Could you check a few things on this model? Use its own coordinates, in mm. A direction names the side the tool comes from. Round coordinates to 2 decimals unless told otherwise and drop trailing zeros. Write each loop counter-clockwise with the first axis right and the second up, starting at its lowest first coordinate (ties: lowest second). Pieces come first, ordered by that corner, then holes. Notation, with made-up numbers: (65, -32) -> (78, -32) arc R13 cw to (78, -16) -> close; hole circle Ø8 at (24.25, 60). An arc over 180 degrees is marked (long way). Return JSON: item names as keys, results as strings.
from build123d import *

# Parameters (mm, degrees)
SKETCH1_W                  = 114
SKETCH1_H                  = 125
BOSS_EXTRUDE1_DEPTH        = 65
SKETCH2_W                  = 111.6
SKETCH2_H                  = 122.6
CUT_EXTRUDE1_DEPTH         = 63.8
SKETCH3_W                  = 44
SKETCH3_H                  = 22
BOSS_EXTRUDE2_DEPTH        = 5
SKETCH4_W                  = 2.65
SKETCH4_H                  = 15
CUT_EXTRUDE2_DEPTH         = 4
SKETCH6_W                  = 2.65
SKETCH6_H                  = 15
CUT_EXTRUDE3_DEPTH         = 4
FILLET1_R                  = 15
FILLET2_R                  = 15
SKETCH9_W                  = 111.6
SKETCH9_H                  = 57.6
SKETCH9_W_2                = 48.6
SKETCH9_H_2                = 48.6
SKETCH9_W_3                = 53.6
SKETCH9_H_3                = 53.6
BOSS_EXTRUDE4_DEPTH        = 9
SKETCH10_W                 = 111.6
SKETCH10_H                 = 56.8
SKETCH10_W_2               = 47
SKETCH10_H_2               = 47
SKETCH10_W_3               = 52
SKETCH10_H_3               = 52
CUT_EXTRUDE5_DEPTH         = 9
SKETCH11_W                 = 4.5
SKETCH11_H                 = 4.5
SKETCH11_H_2               = 56.8
BOSS_EXTRUDE5_DEPTH        = 6
SKETCH12_W                 = 10
SKETCH12_H                 = 5
BOSS_EXTRUDE6_DEPTH        = 5
CHAMFER1_SIZE              = 9
CHAMFER1_SIZE_2            = 5.196152423
CHAMFER1_OF_MIRROR8_SIZE   = 9
CHAMFER1_OF_MIRROR8_SIZE_2 = 5.196152423


with BuildPart() as part:
    # Sketch1 → Boss-Extrude1 (new body)
    with BuildSketch(Plane(origin=(0, 0, 0), x_dir=(1, 0, 0), z_dir=(0, 1, 0))):
        Rectangle(SKETCH1_W, SKETCH1_H)
    extrude(amount=BOSS_EXTRUDE1_DEPTH)

    # Sketch2 → Cut-Extrude1 (cut)
    with BuildSketch(Plane(origin=(0, 65, 0), x_dir=(1, 0, 0), z_dir=(0, 1, 0))):
        Rectangle(SKETCH2_W, SKETCH2_H)
    extrude(amount=-CUT_EXTRUDE1_DEPTH, mode=Mode.SUBTRACT)

    # Sketch3 → Boss-Extrude2 (add)
    with BuildSketch(Plane(origin=(57, 0, 0), x_dir=(0, 0, -1), z_dir=(1, 0, 0))):
        with Locations((-17.5, 44)):
            Rectangle(SKETCH3_W, SKETCH3_H)
    boss_extrude2 = extrude(amount=BOSS_EXTRUDE2_DEPTH)

    # Sketch4 → Cut-Extrude2 (cut)
    with BuildSketch(Plane.XY.offset(39.5)):
        with Locations((58.325, 40.5)):
            Rectangle(SKETCH4_W, SKETCH4_H)
    cut_extrude2 = extrude(amount=-CUT_EXTRUDE2_DEPTH, mode=Mode.SUBTRACT)

    # Sketch6 → Cut-Extrude3 (cut)
    with BuildSketch(Plane(origin=(0, 0, -4.5), x_dir=(-1, 0, 0), z_dir=(0, 0, -1))):
        with Locations((-58.325, 40.5)):
            Rectangle(SKETCH6_W, SKETCH6_H)
    cut_extrude3 = extrude(amount=-CUT_EXTRUDE3_DEPTH, mode=Mode.SUBTRACT)

    # Mirror5: Boss-Extrude2 across plane
    add(boss_extrude2.mirror(Plane(origin=(0, 0, 0), x_dir=(0, 0, 1), z_dir=(1, 0, 0))))

    # Mirror6: Cut-Extrude2 across plane
    add(cut_extrude2.mirror(Plane(origin=(0, 0, 0), x_dir=(0, 0, 1), z_dir=(1, 0, 0))), mode=Mode.SUBTRACT)

    # Mirror7: Cut-Extrude3 across plane
    add(cut_extrude3.mirror(Plane(origin=(0, 0, 0), x_dir=(0, 0, 1), z_dir=(1, 0, 0))), mode=Mode.SUBTRACT)

    # Fillet1
    # the kernel refuses this fillet: 15 mm, written as the material it takes off along each edge
    with BuildSketch(Plane(origin=(62, 33, -32.450849719), x_dir=(-1, 0, 0), z_dir=(0, 0, 1))) as fillet1_piece_1:
        with BuildLine():
            CenterArc((15, -11.180339887), FILLET1_R, 131.810314896, 48.189685104)
            Line((0, -11.180339887), (-0.3, -11.180339887))
            Line((-0.3, -11.180339887), (-0.3, 0))
            Line((-0.3, 0), (0, 0.3))
            ThreePointArc((0, 0.3), (2.5, 0.3), (4.8, 0.223606798))
            Line((4.8, 0.223606798), (5, 0))
        make_face()
    extrude(amount=99.901699437, mode=Mode.SUBTRACT)

    # Fillet2
    # the kernel refuses this fillet: 15 mm, written as the material it takes off along each edge
    with BuildSketch(Plane(origin=(-62, 33, -32.450849719), x_dir=(1, 0, 0), z_dir=(0, 0, 1))) as fillet2_piece_1:
        with BuildLine():
            CenterArc((15, 11.180339887), FILLET2_R, 180, 48.189685104)
            Line((0, 11.180339887), (-0.3, 11.180339887))
            Line((-0.3, 11.180339887), (-0.3, 0))
            Line((-0.3, 0), (0, -0.3))
            ThreePointArc((0, -0.3), (2.5, -0.3), (4.8, -0.223606798))
            Line((4.8, -0.223606798), (5, 0))
        make_face()
    extrude(amount=99.901699437, mode=Mode.SUBTRACT)

    # Sketch9 → Boss-Extrude4 (add)
    with BuildSketch(Plane(origin=(0, 1.2, 0), x_dir=(1, 0, 0), z_dir=(0, 1, 0))):
        with Locations((0, 32.5)):
            Rectangle(SKETCH9_W, SKETCH9_H)
        with Locations((-27.5, -33)):
            Rectangle(SKETCH9_W_2, SKETCH9_H_2)
        with Locations((25, -30.5)):
            Rectangle(SKETCH9_W_3, SKETCH9_H_3)
    extrude(amount=BOSS_EXTRUDE4_DEPTH)

    # Sketch10 → Cut-Extrude5 (cut)
    with BuildSketch(Plane(origin=(0, 10.2, 0), x_dir=(1, 0, 0), z_dir=(0, 1, 0))):
        with Locations((0, 32.9)):
            Rectangle(SKETCH10_W, SKETCH10_H)
        with Locations((-27.5, -33)):
            Rectangle(SKETCH10_W_2, SKETCH10_H_2)
        with Locations((25, -30.5)):
            Rectangle(SKETCH10_W_3, SKETCH10_H_3)
    extrude(amount=-CUT_EXTRUDE5_DEPTH, mode=Mode.SUBTRACT)

    # Sketch11 → Boss-Extrude5 (add)
    with BuildSketch(Plane(origin=(0, 1.2, 0), x_dir=(1, 0, 0), z_dir=(0, 1, 0))):
        with Locations((-53.55, 59.05)):
            Rectangle(SKETCH11_W, SKETCH11_H)
        with Locations((-53.55, 6.75)):
            Rectangle(SKETCH11_W, SKETCH11_H)
        with Locations((53.55, 32.9)):
            Rectangle(SKETCH11_W, SKETCH11_H_2)
        with Locations((-48.75, -11.75)):
            Rectangle(SKETCH11_W, SKETCH11_H)
        with Locations((1.25, -6.75)):
            Rectangle(SKETCH11_W, SKETCH11_H)
        with Locations((-6.25, -11.75)):
            Rectangle(SKETCH11_W, SKETCH11_H)
        with Locations((48.75, -6.75)):
            Rectangle(SKETCH11_W, SKETCH11_H)
        with Locations((-48.75, -54.25)):
            Rectangle(SKETCH11_W, SKETCH11_H)
        with Locations((1.25, -54.25)):
            Rectangle(SKETCH11_W, SKETCH11_H)
        with Locations((-6.25, -54.25)):
            Rectangle(SKETCH11_W, SKETCH11_H)
        with Locations((48.75, -54.25)):
            Rectangle(SKETCH11_W, SKETCH11_H)
        with Locations((0, 32.9)):
            Rectangle(SKETCH11_W, SKETCH11_H)
    extrude(amount=BOSS_EXTRUDE5_DEPTH)

    # Sketch12 → Boss-Extrude6 (add)
    with BuildSketch(Plane.ZY.offset(-55.8)):
        with Locations((-36.3, 34.7)):
            Rectangle(SKETCH12_W, SKETCH12_H)
        with Locations((36.3, 34.7)):
            Rectangle(SKETCH12_W, SKETCH12_H)
    boss_extrude6 = extrude(amount=BOSS_EXTRUDE6_DEPTH)

    # Chamfer1
    # the kernel refuses this chamfer: 9, 5.196152423 mm, written as the material it adds along each edge
    with BuildSketch(Plane(origin=(55.8, 32.2, 41.3), x_dir=(0.019326765612700678, -0.999813220622208, 0), z_dir=(0, 0, -1))) as chamfer1_piece_1_section:
        Polygon((CHAMFER1_SIZE * 0.999813220622, CHAMFER1_SIZE * 0.0193267656127), (-CHAMFER1_SIZE_2 * 0.0193267656116, CHAMFER1_SIZE_2 * 0.999813220566), (0, 0), align=None)
    chamfer1_piece_1 = extrude(amount=10, mode=Mode.PRIVATE)
    chamfer1_piece_1 = split(chamfer1_piece_1, bisect_by=Plane(origin=(50.8, 29.159896695, 36.3), z_dir=(1, 0, 0)), keep=Keep.TOP, mode=Mode.PRIVATE)
    add(chamfer1_piece_1)
    with BuildSketch(Plane(origin=(55.8, 32.2, -31.3), x_dir=(0.019326765612700678, -0.999813220622208, 0), z_dir=(0, 0, -1))) as chamfer1_piece_2_section:
        Polygon((CHAMFER1_SIZE * 0.999813220622, CHAMFER1_SIZE * 0.0193267656127), (-CHAMFER1_SIZE_2 * 0.0193267656116, CHAMFER1_SIZE_2 * 0.999813220566), (0, 0), align=None)
    chamfer1_piece_2 = extrude(amount=10, mode=Mode.PRIVATE)
    chamfer1_piece_2 = split(chamfer1_piece_2, bisect_by=Plane(origin=(50.8, 29.159896695, -36.3), z_dir=(1, 0, 0)), keep=Keep.TOP, mode=Mode.PRIVATE)
    add(chamfer1_piece_2)

    # Mirror8: Boss-Extrude6 across plane
    add(boss_extrude6.mirror(Plane(origin=(0, 0, 0), x_dir=(0, 0, 1), z_dir=(1, 0, 0))))

    # Chamfer1 of Mirror8
    # the kernel refuses this chamfer: 9, 5.196152423 mm, written as the material it adds along each edge
    with BuildSketch(Plane(origin=(-55.8, 32.2, 41.3), x_dir=(-0.01932676561270296, -0.9998132206222078, 0), z_dir=(0, 0, -1))) as chamfer1_of_mirror8_piece_1_section:
        Polygon((CHAMFER1_OF_MIRROR8_SIZE * 0.999813220622, -CHAMFER1_OF_MIRROR8_SIZE * 0.0193267656127), (-CHAMFER1_OF_MIRROR8_SIZE_2 * 0.0193267656116, -CHAMFER1_OF_MIRROR8_SIZE_2 * 0.999813220566), (0, 0), align=None)
    chamfer1_of_mirror8_piece_1 = extrude(amount=10, mode=Mode.PRIVATE)
    chamfer1_of_mirror8_piece_1 = split(chamfer1_of_mirror8_piece_1, bisect_by=Plane(origin=(-50.8, 29.159896695, 36.3), z_dir=(-1, 0, 0)), keep=Keep.TOP, mode=Mode.PRIVATE)
    add(chamfer1_of_mirror8_piece_1)
    with BuildSketch(Plane(origin=(-55.8, 32.2, -31.3), x_dir=(-0.01932676561270296, -0.9998132206222078, 0), z_dir=(0, 0, -1))) as chamfer1_of_mirror8_piece_2_section:
        Polygon((CHAMFER1_OF_MIRROR8_SIZE * 0.999813220622, -CHAMFER1_OF_MIRROR8_SIZE * 0.0193267656127), (-CHAMFER1_OF_MIRROR8_SIZE_2 * 0.0193267656116, -CHAMFER1_OF_MIRROR8_SIZE_2 * 0.999813220566), (0, 0), align=None)
    chamfer1_of_mirror8_piece_2 = extrude(amount=10, mode=Mode.PRIVATE)
    chamfer1_of_mirror8_piece_2 = split(chamfer1_of_mirror8_piece_2, bisect_by=Plane(origin=(-50.8, 29.159896695, -36.3), z_dir=(-1, 0, 0)), keep=Keep.TOP, mode=Mode.PRIVATE)
    add(chamfer1_of_mirror8_piece_2)


solid = part.part
1) For faces 1 (the face through (46.5, 4, 54)), 2 (the face through (53.335, 27.47, 36.37)), 3 (the face through (-59.65, 42, -3)), which set-ups out of +Z, -Z, +X, -X, +Y, -Y let a thin tool reach every point of the face, with its end or its side?
Return value:
{"face 1": "+Y", "face 2": "none", "face 3": "-Z, -Y"}
2) I want a section at C-C, the plane z = -28.5. Please give me the cut outline in (x, y), and give its area (3 significant figures).
Return value:
{"outline": "(-57, 0) -> (57, 0) -> (57, 65) -> (55.8, 65) -> (55.8, 7.2) -> (51.3, 7.2) -> (51.3, 1.2) -> (-55.8, 1.2) -> (-55.8, 65) -> (-57, 65) -> close", "area": "317 mm²"}
3) If I drill on probe 1 along Z at (x, y) = (-12, 8.5); probe 2 along Z at (x, y) = (32, 6); probe 3 along X at (y, z) = (10, 32), over which ranges is the centre line in solid material (lowest first)? Write a range as [from, to].
Return value:
{"probe 1": "[-62.5, -61.3], [-4.5, -3.7], [8.7, 9.5], [56.5, 57.3], [61.3, 62.5]", "probe 2": "[-62.5, -61.3], [-4.5, -3.7], [3.7, 4.5], [56.5, 57.3], [61.3, 62.5]", "probe 3": "[-57, -55.8], [-51.8, -51], [-4, -3.2], [-1.8, -1], [51, 51.8], [55.8, 57]"}
4) Will these pins go through, and if not, where does the flat tip stop? pin 1 Ø1.2 at (y, z) = (39.5, -2.5) entering from +X; pin 2 Ø1 at (x, z) = (-39.5, -39) entering from +Y; pin 3 Ø3.5 at (y, z) = (5, 53) entering from +X; pin 4 Ø6 at (x, z) = (37.5, -33) entering from -Y.
Return value:
{"pin 1": "x = 61.43", "pin 2": "y = 1.2", "pin 3": "x = 57", "pin 4": "y = 0"}
5) I want a section at A-A, the plane z = 46.5. Please give me the cut outline in (x, y).
Return value:
{"outline": "(-57, 0) -> (57, 0) -> (57, 65) -> (55.8, 65) -> (55.8, 1.2) -> (51.8, 1.2) -> (51.8, 10.2) -> (51, 10.2) -> (51, 1.2) -> (-1, 1.2) -> (-1, 10.2) -> (-1.8, 10.2) -> (-1.8, 1.2) -> (-3.2, 1.2) -> (-3.2, 10.2) -> (-4, 10.2) -> (-4, 1.2) -> (-51, 1.2) -> (-51, 10.2) -> (-51.8, 10.2) -> (-51.8, 1.2) -> (-55.8, 1.2) -> (-55.8, 65) -> (-57, 65) -> close"}
6) I want a section at B-B, the plane x = -40. Please give me the cut outline in (y, z), and give its area (3 significant figures).
Return value:
{"outline": "(0, -62.5) -> (65, -62.5) -> (65, -61.3) -> (1.2, -61.3) -> (1.2, -4.5) -> (10.2, -4.5) -> (10.2, -3.7) -> (1.2, -3.7) -> (1.2, 8.7) -> (10.2, 8.7) -> (10.2, 9.5) -> (1.2, 9.5) -> (1.2, 56.5) -> (10.2, 56.5) -> (10.2, 57.3) -> (1.2, 57.3) -> (1.2, 61.3) -> (65, 61.3) -> (65, 62.5) -> (0, 62.5) -> close", "area": "325 mm²"}
7) Thinking about a two-plate mould opening in X: for faces 4 (the face through (-59, 55, 18)), 5 (the face through (-6, 4, 52)), which applies, pulls with the +X half, pulls with the -X half, needs draft (parallel to the pull), parting line crosses it, or undercut?
Return value:
{"face 4": "needs draft", "face 5": "undercut"}
8) I want a section at D-D, the plane x = 49. Please give me the cut outline in (y, z), and give its area (3 significant figures).
Return value:
{"outline": "(0, -62.5) -> (65, -62.5) -> (65, -61.3) -> (1.2, -61.3) -> (1.2, -4.5) -> (10.2, -4.5) -> (10.2, -3.7) -> (1.2, -3.7) -> (1.2, 3.7) -> (10.2, 3.7) -> (10.2, 4.5) -> (7.2, 4.5) -> (7.2, 9) -> (1.2, 9) -> (1.2, 52) -> (7.2, 52) -> (7.2, 56.5) -> (10.2, 56.5) -> (10.2, 57.3) -> (1.2, 57.3) -> (1.2, 61.3) -> (65, 61.3) -> (65, 62.5) -> (0, 62.5) -> close", "area": "379 mm²"}
